from build123d import *

# Parameters (mm, degrees)
SKETCH1_W                = 88.9
SKETCH1_H                = 22.225
BOSS_EXTRUDE1_DEPTH      = 2.54
SKETCH2_W                = 99.06
SKETCH2_H                = 32.385
SKETCH2_W_2              = 88.9
SKETCH2_H_2              = 22.225
BOSS_EXTRUDE3_DEPTH      = 34.925
BOSS_EXTRUDE3_DEPTH_BACK = 2.54
SKETCH4_W                = 120.635507722
SKETCH4_H                = 32.385
SKETCH4_W_2              = 88.9
SKETCH4_H_2              = 22.225
BOSS_EXTRUDE4_DEPTH      = 5.08
SKETCH5_W                = 12.7
SKETCH5_H                = 51.435
BOSS_EXTRUDE5_DEPTH      = 6.35
BOSS_EXTRUDE6_DEPTH      = 32.385
SKETCH7_W                = 15.867753861
SKETCH7_H                = 17.145
CUT_EXTRUDE1_DEPTH       = 11.43


with BuildPart() as part:
    # Sketch1 → Boss-Extrude1 (new body)
    with BuildSketch(Plane(origin=(0, 0, 0), x_dir=(1, 0, 0), z_dir=(0, 1, 0))):
        Rectangle(SKETCH1_W, SKETCH1_H)
    extrude(amount=BOSS_EXTRUDE1_DEPTH)

    # Sketch2 → Boss-Extrude3 (add, two sides)
    with BuildSketch(Plane(origin=(0, 2.54, 0), x_dir=(1, 0, 0), z_dir=(0, 1, 0))) as boss_extrude3_sk:
        Rectangle(SKETCH2_W, SKETCH2_H)
        Rectangle(SKETCH2_W_2, SKETCH2_H_2, mode=Mode.SUBTRACT)
    extrude(amount=BOSS_EXTRUDE3_DEPTH)
    extrude(boss_extrude3_sk.sketch, amount=-BOSS_EXTRUDE3_DEPTH_BACK)

    # Sketch4 → Boss-Extrude4 (add)
    with BuildSketch(Plane(origin=(0, 37.465, 0), x_dir=(1, 0, 0), z_dir=(0, 1, 0))):
        Rectangle(SKETCH4_W, SKETCH4_H)
        Rectangle(SKETCH4_W_2, SKETCH4_H_2, mode=Mode.SUBTRACT)
    extrude(amount=BOSS_EXTRUDE4_DEPTH)

    # Sketch5 → Boss-Extrude5 (add)
    with BuildSketch(Plane(origin=(0, 42.545, 0), x_dir=(1, 0, 0), z_dir=(0, 1, 0))):
        with Locations((53.967753861, 0)):
            Rectangle(SKETCH5_W, SKETCH5_H)
        with Locations((-53.967753861, 0)):
            Rectangle(SKETCH5_W, SKETCH5_H)
    extrude(amount=BOSS_EXTRUDE5_DEPTH)

    # Sketch6 → Boss-Extrude6 (add)
    with BuildSketch(Plane(origin=(0, 0, -16.1925), x_dir=(-1, 0, 0), z_dir=(0, 0, -1))):
        Polygon((-49.53, 0), (-60.317753861, 37.465), (-49.53, 37.465), align=None)
        Polygon((49.53, 37.465), (60.317753861, 37.465), (49.53, 0), align=None)
    extrude(amount=-BOSS_EXTRUDE6_DEPTH)

    # Sketch7 → Cut-Extrude1 (cut)
    with BuildSketch(Plane(origin=(0, 48.895, 0), x_dir=(1, 0, 0), z_dir=(0, 1, 0))):
        with Locations((52.383876931, 0)):
            Rectangle(SKETCH7_W, SKETCH7_H)
    extrude(amount=-CUT_EXTRUDE1_DEPTH, mode=Mode.SUBTRACT)


solid = part.part
The model under review builds one solid part; all positions refer to its coordinate system, in mm. A direction names the side the tool comes from. Round coordinates to 2 decimals unless told otherwise and drop trailing zeros. Order: outer loops, then holes, each group sorted by start corner. A loop starts at its lowest first (then second) coordinate and runs counter-clockwise, first axis right, second up. Notation, with made-up numbers: (45.25, 51) -> (72.25, 51) arc R12 ccw to (72.25, 65) -> close; hole circle Ø11 at (84.25, 87). An arc over 180 degrees is marked (long way). Return JSON: item names as keys, results as strings.
1. Take a section at D-D (z = -6.5). Write out the cut boundary in (x, y) (3 decimals), then the cut area to 3 significant figures.
Answer block:
{"outline": "(-60.318, 37.465) -> (-49.53, 0) -> (49.53, 0) -> (60.318, 37.465) -> (44.45, 37.465) -> (44.45, 2.54) -> (-44.45, 2.54) -> (-44.45, 42.545) -> (-47.618, 42.545) -> (-47.618, 48.895) -> (-60.318, 48.895) -> close", "area": "1,170 mm²"}
2. For L1, parallel to Z at x = -32.5, y = 8; L2, parallel to Z at x = -52, y = 29; L3, parallel to X at y = 40, z = 4.5, list the stretches that pass through material, from the lowest coordinate up. Write a range as [from, to].
Answer block:
{"L1": "z = [-16.19, -11.11], [11.11, 16.19]", "L2": "z = [-16.19, 16.19]", "L3": "x = [-60.32, -44.45]"}
3. Take a section at B-B (x = 26.5). Write out the cut boundary in (y, z) (1 decimal), then the cut area to 3 significant figures.
Answer block:
{"outline": "(0, -16.2) -> (42.5, -16.2) -> (42.5, -11.1) -> (2.5, -11.1) -> (2.5, 11.1) -> (42.5, 11.1) -> (42.5, 16.2) -> (0, 16.2) -> close", "area": "489 mm²"}
4. Take a section at C-C (y = 36). Write out the cut boundary in (x, z).
Answer block:
{"outline": "(-59.9, -16.19) -> (59.9, -16.19) -> (59.9, 16.19) -> (-59.9, 16.19) -> close; hole (-44.45, -11.11) -> (44.45, -11.11) -> (44.45, 11.11) -> (-44.45, 11.11) -> close"}
5. For faces 4 (the face through (52, 37.465, 0)), 5 (the face through (-1, 22, 11.112)), 6 (the face through (-54, 42.545, -21)), 7 (the face through (-55, 19, 0)), 8 (the face through (-1, 22, 16.192)), list the 3-axis set-ups (+Z, -Z, +X, -X, +Y, -Y) from which the entire face can be reached by the end or side of a thin tool; tool diameter is ignored.
Answer block:
{"face 4": "+X, +Y", "face 5": "+Y", "face 6": "-Z, +X, -X, -Y", "face 7": "+Z, -Z, -X, -Y", "face 8": "+Z, +X, -X, -Y"}
6. Insertion check: P1, Ø24.5, axis at y = 24, z = 5, coming from the -X side; P2, Ø1, axis at y = 29.5, z = 0.5, coming from the -X side; P3, Ø8, axis at x = -46, z = 7, coming from the -Y side; P4, Ø11, axis at x = -21.5, z = -0.5, coming from the +Y side. Each pin has a flat end and moves straight along its axis. Give the tip position at first contact, or say it passes through.
Answer block:
{"P1": "stops at x = -59.97", "P2": "stops at x = -58.17", "P3": "stops at y = 0", "P4": "stops at y = 2.54"}
7. The part is to be moulded in two halves that separate along X. For faces 1 (the face through (-47.618, 46, 0)), 2 (the face through (54, 42.545, 21)), 3 (the face through (60.318, 44, -15)), say which applies: +X half, -X half, draft (parallel to the pull), parting line (faces both ways), or undercut.
Answer block:
{"face 1": "undercut", "face 2": "draft", "face 3": "+X half"}
8. Take a section at A-A (z = 22). Write out the cut boundary in (x, y) (3 decimals).
Answer block:
{"outline": "(-60.318, 42.545) -> (-47.618, 42.545) -> (-47.618, 48.895) -> (-60.318, 48.895) -> close; (47.618, 42.545) -> (60.318, 42.545) -> (60.318, 48.895) -> (47.618, 48.895) -> close"}
